Build history of the part. All positions in model axes, mm. Face numbers are marked on the shaded views. A direction names the side the tool comes from. Give positions to 0.01 mm unless a question says otherwise; leave off trailing zeros. Order: outer loops, then holes, each group sorted by start corner. A loop starts at its lowest first (then second) coordinate and runs counter-clockwise, first axis right, second up. Notation, with made-up numbers: (-10.5, 5) -> (9.5, 5) arc R21 ccw to (9.5, 29) -> close; hole circle Ø3 at (-25, 40.25). An arc over 180 degrees is marked (long way). Use a Markdown table: item, result. Add a question column.
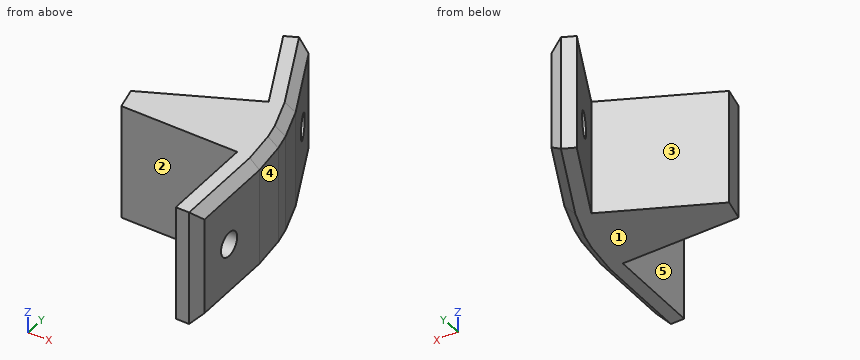
```python
from build123d import *

# Parameters (mm, degrees)
BOSS_EXTRU_1_DEPTH      = 20
ESQUISSE2_W             = 20
ESQUISSE2_H             = 20
BOSS_EXTRU_2_DEPTH      = 2
ESQUISSE3_W             = 20
ESQUISSE3_H             = 20
BOSS_EXTRU_3_DEPTH      = 2
ESQUISSE4_W             = 20
ESQUISSE4_H             = 8.998042174
BOSS_EXTRU_4_DEPTH      = 4
BOSS_EXTRU_5_DEPTH      = 20
CHANFREIN1_SIZE         = 3
CHANFREIN2_SIZE         = 1.6
ESQUISSE7_R             = 2.1
ENL_V_MAT_EXTRU_1_DEPTH = 13.855900094
ESQUISSE8_R             = 2.1
ENL_V_MAT_EXTRU_2_DEPTH = 4.897480259
BOSS_EXTRU_6_DEPTH      = 20


with BuildPart() as part:
    # Esquisse1 → Boss.-Extru.1 (new body)
    with BuildSketch(Plane.XY):
        Polygon((0, 0), (20, 0), (17.975880926, 8.767422936), align=None)
    extrude(amount=BOSS_EXTRU_1_DEPTH)

    # Esquisse2 → Boss.-Extru.2 (add)
    with BuildSketch(Plane(origin=(0, 0, 0), x_dir=(0.898794046, 0.438371147, 0), z_dir=(-0.438371147, 0.898794046, 0))):
        with Locations((10, -10)):
            Rectangle(ESQUISSE2_W, ESQUISSE2_H)
    extrude(amount=BOSS_EXTRU_2_DEPTH)

    # Esquisse3 → Boss.-Extru.3 (add)
    with BuildSketch(Plane.XZ):
        with Locations((10, 10)):
            Rectangle(ESQUISSE3_W, ESQUISSE3_H)
    extrude(amount=BOSS_EXTRU_3_DEPTH)

    # Esquisse4 → Boss.-Extru.4 (add)
    with BuildSketch(Plane(origin=(18.987940463, 4.383711468, 0), x_dir=(0, 0, -1), z_dir=(0.974370065, 0.224951054, 0))):
        with Locations((-10, 0)):
            Rectangle(ESQUISSE4_W, ESQUISSE4_H)
    extrude(amount=BOSS_EXTRU_4_DEPTH)

    # Esquisse5 → Boss.-Extru.5 (add)
    with BuildSketch(Plane.XY.offset(20)):
        Polygon((17.099138632, 10.565011028), (10.085200284, 24.945715769), (13.588232336, 26.65425866), (21.873361185, 9.667227153), (17.975880926, 8.767422936), align=None)
        Polygon((20, 0), (20, -2), (20, -18), (23.897480259, -18), (23.897480259, 0.899804217), align=None)
    extrude(amount=-BOSS_EXTRU_5_DEPTH)

    # Chanfrein1
    chanfrein1_edges = [part.edges().sort_by_distance(p)[0] for p in [
        (23.897480259, 0.899804217, 10),
        (21.873361185, 9.667227153, 10),
    ]]
    chamfer(chanfrein1_edges, length=CHANFREIN1_SIZE)

    # Chanfrein2
    chanfrein2_edges = [part.edges().sort_by_distance(p)[0] for p in [
        (13.588232336, 26.65425866, 10),
        (23.897480259, -10.050097891, 0),
        (23.897480259, -18, 10),
        (23.897480259, -10.050097891, 20),
        (22.885420722, 5.283515685, 20),
        (22.885420722, 5.283515685, 0),
        (17.073240041, 19.508933976, 0),
        (21.553231046, 9.553863125, 0),
        (23.560053678, 0.861359315, 0),
        (17.073240041, 19.508933976, 20),
        (21.553231046, 9.553863125, 20),
        (23.560053678, 0.861359315, 20),
    ]]
    chamfer(chanfrein2_edges, length=CHANFREIN2_SIZE)

    # Esquisse7 → Enlèv. mat.-Extru.1 (cut, through all)
    with BuildSketch(Plane(origin=(17.975880926, 8.767422936, 0), x_dir=(0, 0, 1), z_dir=(-0.898794046, -0.438371147, 0))):
        with Locations((10, 10)):
            Circle(ESQUISSE7_R)
    extrude(amount=-ENL_V_MAT_EXTRU_1_DEPTH, mode=Mode.SUBTRACT)

    # Esquisse8 → Enlèv. mat.-Extru.2 (cut, through all)
    with BuildSketch(Plane.ZY.offset(-20)):
        with Locations((10, -10)):
            Circle(ESQUISSE8_R)
    extrude(amount=-ENL_V_MAT_EXTRU_2_DEPTH, mode=Mode.SUBTRACT)

    # Esquisse9 → Boss.-Extru.6 (add)
    with BuildSketch(Plane.XY.offset(20)):
        Polygon((-0.876742294, 1.797588093), (0, 0), (0, -2), align=None)
    extrude(amount=-BOSS_EXTRU_6_DEPTH)


solid = part.part
```
(1) Mould opens along Y. For the marked faces 1, 2 and 3 say: released by +Y, released by -Y, zero draft, split by the parting line, or undercut.
(2) Pin check, flat tips, straight feed: pin 1 Ø5 at (y, z) = (-6.5, 10) entering from -X; pin 2 Ø4 at (y, z) = (12, 3.5) entering from -X; pin 3 Ø8 at (y, z) = (0, 4.5) entering from +X; pin 4 Ø3 at (x, z) = (3.5, 6.5) entering from +Y. Stop position of each tip, or through.
(3) Band-saw the part on A-A on y = -10. Give the cut face in (x, z).
(4) Tool access for the marked faces 4 and 5: list every direction of +Z, -Z, +X, -X, +Y, -Y with a clear straight run to the whole face (end or side of a thin tool).
(5) Wall check: probe 1 along X at (y, z) = (-15, 17.5); probe 2 along Y at (x, z) = (13.25, 14); probe 3 along Y at (x, z) = (10.75, 8.5). Give the ranges that are in metal, low to high.
(6) Band-saw the part on B-B on z = 14.25. Give the cut face in (x, y).
(7) Band-saw the part on D-D on y = 15. Give the cut face in (x, z), plus the area to 3 significant figures.
(8) Band-saw the part on C-C on z = 10. Give the cut face in (x, y), plus the area to 3 significant figures.
Response:
| question | item | result |
|---|---|---|
| 1 | face 1 | zero draft |
| 1 | face 2 | released by -Y |
| 1 | face 3 | undercut |
| 2 | pin 1 | stops at x = 20 |
| 2 | pin 2 | stops at x = 15.42 |
| 2 | pin 3 | stops at x = 23.9 |
| 2 | pin 4 | stops at y = 4.66 |
| 3 | outline | (20, 0) -> (22.3, 0) -> (23.9, 1.6) -> (23.9, 7.9) -> (20, 7.9) -> close; (20, 12.1) -> (23.9, 12.1) -> (23.9, 18.4) -> (22.3, 20) -> (20, 20) -> close |
| 4 | face 4 | +Z, -Z, +X, +Y |
| 4 | face 5 | +Z, -Z, -X, -Y |
| 5 | probe 1 | x = 20 to 23.9 |
| 5 | probe 2 | y = -2 to 8.69, 18.46 to 25.57 |
| 5 | probe 3 | y = -2 to 7.47, 23.58 to 25.27 |
| 6 | outline | (-0.88, 1.8) -> (0, -2) -> (20, -2) -> (20, -18) -> (22.3, -18) -> (23.9, -16.4) -> (23.9, -2.1) -> (23.22, 3.82) -> (22.55, 6.74) -> (20.56, 12.36) -> (14.29, 25.22) -> (12.15, 25.95) -> (10.09, 24.95) -> (17.1, 10.57) -> close |
| 7 | outline | (14.94, 0) -> (17.49, 0) -> (19.27, 1.6) -> (19.27, 18.4) -> (17.49, 20) -> (14.94, 20) -> close |
| 7 | area | 83.9 mm² |
| 8 | outline | (-0.88, 1.8) -> (0, -2) -> (20, -2) -> (20, -7.9) -> (23.9, -7.9) -> (23.9, -2.1) -> (23.22, 3.82) -> (22.55, 6.74) -> (20.56, 12.36) -> (18.02, 17.58) -> (14.51, 15.87) -> (17.1, 10.57) -> close; (10.09, 24.95) -> (12.67, 19.64) -> (16.17, 21.35) -> (14.29, 25.22) -> (12.15, 25.95) -> close; (20, -18) -> (22.3, -18) -> (23.9, -16.4) -> (23.9, -12.1) -> (20, -12.1) -> close |
| 8 | area | 311 mm² |
